Can you work these out from the drawing? Everything is in mm from the part's minimum corner. A direction names the side the tool comes from. Give positions to 0.01 mm unless a question says otherwise; leave off trailing zeros. Order: outer loops, then holes, each group sorted by start corner. A loop starts at its lowest first (then second) coordinate and runs counter-clockwise, first axis right, second up. Notation, with made-up numbers: M 14.25,50 L 18.25,50 A12 cw 18.25,65 Z; hole C 77.25,-17.75 d7. An arc over 180 degrees is marked long. Answer as a JSON object with one key per item and string values.
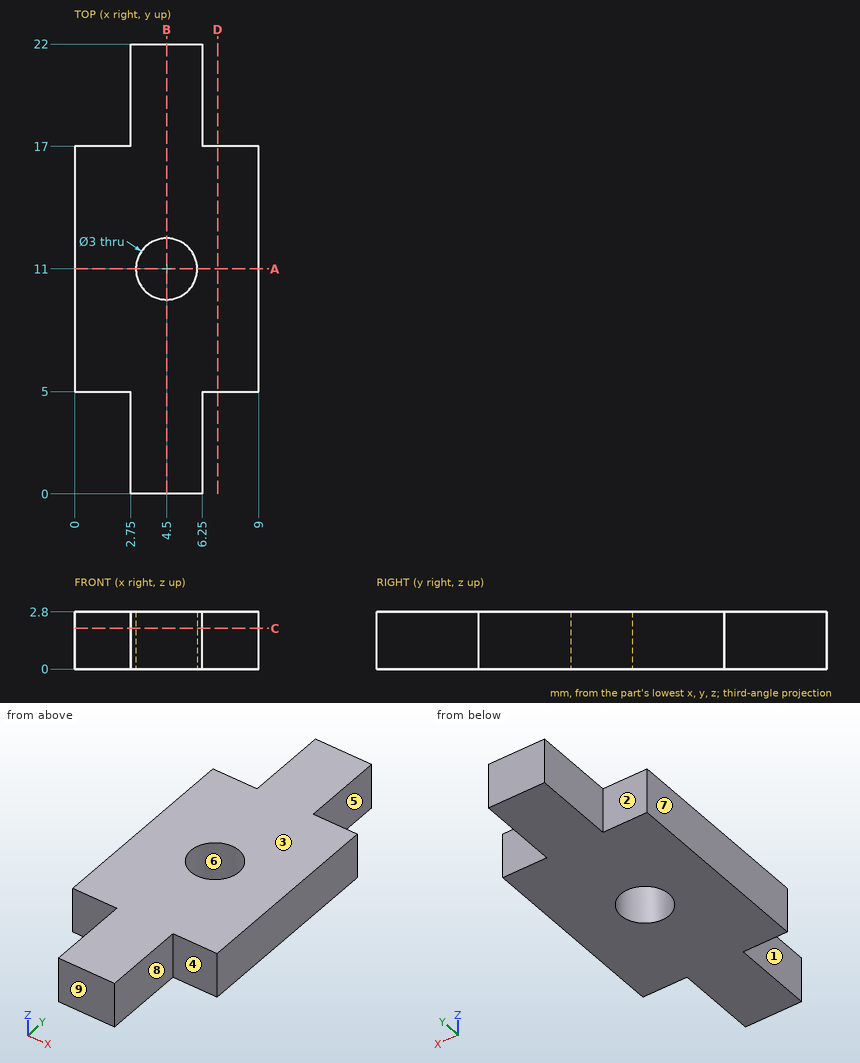
1) Thinking about a two-plate mould opening in X: for the marked faces 6, 7, 8 and 9, which applies, pulls with the +X half, pulls with the -X half, needs draft (parallel to the pull), parting line crosses it, or undercut?
Results found:
{"face 6": "undercut", "face 7": "pulls with the -X half", "face 8": "pulls with the +X half", "face 9": "needs draft"}
2) For the marked faces 1, 2, 3, 4 and 5, which set-ups out of +Z, -Z, +X, -X, +Y, -Y let a thin tool reach every point of the face, with its end or its side?
Results found:
{"face 1": "+Z, -Z, -X, -Y", "face 2": "+Z, -Z, -X, +Y", "face 3": "+Z, +X, -X, +Y, -Y", "face 4": "+Z, -Z, +X, -Y", "face 5": "+Z, -Z, +X, +Y"}
3) I want a section at C-C on z = 2. Write out the boundary of the cut face in (x, y), and give its area (3 significant figures).
Results found:
{"outline": "M 0,5 L 2.75,5 L 2.75,0 L 6.25,0 L 6.25,5 L 9,5 L 9,17 L 6.25,17 L 6.25,22 L 2.75,22 L 2.75,17 L 0,17 Z; hole C 4.5,11 d3", "area": "136 mm²"}
4) I want a section at A-A on y = 11. Write out the boundary of the cut face in (x, z), and give its area (3 significant figures).
Results found:
{"outline": "M 0,0 L 3,0 L 3,2.8 L 0,2.8 Z; M 6,0 L 9,0 L 9,2.8 L 6,2.8 Z", "area": "16.8 mm²"}
5) I want a section at B-B on x = 4.5. Write out the boundary of the cut face in (y, z).
Results found:
{"outline": "M 0,0 L 9.5,0 L 9.5,2.8 L 0,2.8 Z; M 12.5,0 L 22,0 L 22,2.8 L 12.5,2.8 Z"}
6) I want a section at D-D on x = 7. Write out the boundary of the cut face in (y, z), and give its area (3 significant figures).
Results found:
{"outline": "M 5,0 L 17,0 L 17,2.8 L 5,2.8 Z", "area": "33.6 mm²"}
7) I'm going to push flat-ended pins straight in: pin 1 Ø1.4 at (y, z) = (3, 1) entering from -X; pin 2 Ø4 at (x, y) = (4.5, 11) entering from -Z; pin 3 Ø1.4 at (y, z) = (3, 2) entering from +X. Where does each tip first touch, or does it pass through?
Results found:
{"pin 1": "stops at x = 2.75", "pin 2": "stops at z = 0", "pin 3": "stops at x = 6.25"}
8) I need wall thicknesses on L1, parallel to Y at x = 4.5, z = 1.55; L2, parallel to Y at x = 7, z = 2; L3, parallel to Y at x = 3.25, z = 0.3. Which ranges of each line are inside material? Lowest first, please.
Results found:
{"L1": "y = 0 to 9.5, 12.5 to 22", "L2": "y = 5 to 17", "L3": "y = 0 to 10.17, 11.83 to 22"}
